Part model, mm, in its own coordinate system. A direction names the side the tool comes from. Coordinates: 2 decimals unless noted, no trailing zeros. Loops run counter-clockwise (first coordinate to the right, second up) from the corner with the lowest first, then second, coordinate; pieces in that order, holes last. Notation, with made-up numbers: (-31.5, 68) - (-23.5, 68) arc R32 ccw to (-23.5, 106) - close; hole circle Ø3 at (31.25, 55.5). An arc over 180 degrees is marked (long way). Use a Markdown table: item, result. Add a question column.
1. Band-saw the part on A-A, the plane y = -11. Give the cut face in (x, z).
2. Band-saw the part on B-B, the plane x = 8.5. Count the separate pieces of the cut face and the enclosed holes in it, plus the area to 3 significant figures.
3. Pull direction Z, two halves, no side cores. Call faces 4 (the flat face through (4, -46.7, 0)), 5 (the cylindrical face through (-19.458, -53.208, -6.128)), 6 (the flat face through (14, -59.9, 14)): pulls with the +Z half, pulls with the -Z half, needs draft (parallel to the pull), parting line crosses it, or undercut.
4. Wall check: probe 1 along Z at (x, y) = (0, -55.5); probe 2 along Y at (x, z) = (-11.5, -14.5); probe 3 along X at (y, z) = (-54.5, 17.5). Give the ranges that are in metal, low to high. Write a range as [from, to].
5. Drop flat-ended pins along their axis: pin 1 (2.5 mm diameter, centred on x = 14.5, z = 8, fed in from -Y); pin 2 (2 mm diameter, centred on x = 11, z = 15.5, fed in from +Y); pin 3 (1 mm diameter, centred on x = -18, y = -55.5, fed in from +Z). Give the stop position or say it passes through.
6. Band-saw the part on D-D, the plane y = -42. Give the cut face in (x, z).
7. 3-axis set-ups, long thin cutter, end or side, ignore diameter. For faces 1 (the flat face through (0, -47.4, 18)), 2 (the cylindrical face through (0, -62, 2)), 3 (the cylindrical face through (8.87, -45.94, 6.94)): which of +Z, -Z, +X, -X, +Y, -Y reach the whole face in a straight line?
from build123d import *

# Parameters (mm, degrees)
SKETCH2_R          = 4.25
CUT_EXTRUDE1_DEPTH = 54.622383424
CHAMFER1_SIZE      = 0.5
CIRPATTERN1_START  = -59.4
CIRPATTERN1_DEPTH  = 12


# Read off the part's stored shape, not the designer's step: CirPattern1
with BuildPart() as part:
    # Sketch1 → Revolve1 (revolve)
    with BuildSketch(Plane.XY, mode=Mode.PRIVATE) as revolve1_sk:
        with BuildLine():
            Line((0, 0), (0, -77.5))
            Line((0, -77.5), (2, -77.5))
            Line((2, -77.5), (2, -46.7))
            Line((2, -46.7), (18.9, -46.7))
            Line((18.9, -46.7), (18.9, -59.9))
            Line((18.9, -59.9), (20.4, -59.9))
            Line((20.4, -59.9), (20.4, -46.7))
            ThreePointArc((20.4, -46.7), (19.960660172, -45.639339828), (18.9, -45.2))
            Line((18.9, -45.2), (6, -45.2))
            ThreePointArc((6, -45.2), (5.292893219, -44.907106781), (5, -44.2))
            Line((5, -44.2), (5, -39.7))
            ThreePointArc((5, -39.7), (4.853553391, -39.346446609), (4.5, -39.2))
            Line((4.5, -39.2), (2, -39.2))
            Line((2, -39.2), (2, 0))
            Line((2, 0), (0, 0))
        make_face()
    revolve(revolve1_sk.sketch.rotate(Axis((0, 0, 0), (0, -1, 0)), 180), axis=Axis((0, 0, 0), (0, -1, 0)))

    # Sketch2 → Cut-Extrude1 (cut, through all)
    with BuildSketch(Plane(origin=(0, -45.2, 0), x_dir=(1, 0, 0), z_dir=(0, 1, 0))):
        with Locations(Location((5.5, 9.526279442, 0), (0, 0, 180))):
            Circle(SKETCH2_R)
        with Locations(Location((11, 0, 0), (0, 0, 180))):
            Circle(SKETCH2_R)
        with Locations(Location((5.5, -9.526279442, 0), (0, 0, 180))):
            Circle(SKETCH2_R)
        with Locations(Location((-5.5, -9.526279442, 0), (0, 0, 180))):
            Circle(SKETCH2_R)
        with Locations(Location((-11, 0, 0), (0, 0, 180))):
            Circle(SKETCH2_R)
        with Locations(Location((-5.5, 9.526279442, 0), (0, 0, 180))):
            Circle(SKETCH2_R)
    extrude(amount=-CUT_EXTRUDE1_DEPTH, mode=Mode.SUBTRACT)

    # Chamfer1
    chamfer1_edges = [part.edges().sort_by_distance(p)[0] for p in [
        (2, 0, 0),
        (2, -77.5, 0),
    ]]
    chamfer(chamfer1_edges, length=CHAMFER1_SIZE)

    # CirPattern1 outline → CirPattern1 (add)
    with BuildSketch(Plane(origin=(0, 0, 0), x_dir=(1, 0, 0), z_dir=(0, 1, 0)).offset(CIRPATTERN1_START)):
        with BuildLine():
            ThreePointArc((-3.9, -18.493242009), (0, -18.9), (3.9, -18.493242009))
            Line((3.9, -18.493242009), (3.9, -17.3))
            Line((3.9, -17.3), (-3.9, -17.3))
            Line((-3.9, -17.3), (-3.9, -18.493242009))
        make_face()
        with BuildLine():
            Line((5.272500925, -16.932239485), (5.86912193, -17.965617378))
            ThreePointArc((5.86912193, -17.965617378), (9.45, -16.367880131), (12.624120079, -14.065617378))
            Line((12.624120079, -14.065617378), (12.027499075, -13.032239485))
            Line((12.027499075, -13.032239485), (5.272500925, -16.932239485))
        make_face()
        with BuildLine():
            ThreePointArc((-12.624120079, -14.065617378), (-9.45, -16.367880131), (-5.86912193, -17.965617378))
            Line((-5.86912193, -17.965617378), (-5.272500925, -16.932239485))
            Line((-5.272500925, -16.932239485), (-12.027499075, -13.032239485))
            Line((-12.027499075, -13.032239485), (-12.624120079, -14.065617378))
        make_face()
        with BuildLine():
            Line((13.032239485, -12.027499075), (14.065617378, -12.624120079))
            ThreePointArc((14.065617378, -12.624120079), (16.367880131, -9.45), (17.965617378, -5.86912193))
            Line((17.965617378, -5.86912193), (16.932239485, -5.272500925))
            Line((16.932239485, -5.272500925), (13.032239485, -12.027499075))
        make_face()
        with BuildLine():
            ThreePointArc((-17.965617378, -5.86912193), (-16.367880131, -9.45), (-14.065617378, -12.624120079))
            Line((-14.065617378, -12.624120079), (-13.032239485, -12.027499075))
            Line((-13.032239485, -12.027499075), (-16.932239485, -5.272500925))
            Line((-16.932239485, -5.272500925), (-17.965617378, -5.86912193))
        make_face()
        with BuildLine():
            Line((17.3, -3.9), (18.493242009, -3.9))
            ThreePointArc((18.493242009, -3.9), (18.9, 0), (18.493242009, 3.9))
            Line((18.493242009, 3.9), (17.3, 3.9))
            Line((17.3, 3.9), (17.3, -3.9))
        make_face()
        with BuildLine():
            ThreePointArc((-18.493242009, 3.9), (-18.9, 0), (-18.493242009, -3.9))
            Line((-18.493242009, -3.9), (-17.3, -3.9))
            Line((-17.3, -3.9), (-17.3, 3.9))
            Line((-17.3, 3.9), (-18.493242009, 3.9))
        make_face()
        with BuildLine():
            ThreePointArc((-14.065617378, 12.624120079), (-16.367880131, 9.45), (-17.965617378, 5.86912193))
            Line((-17.965617378, 5.86912193), (-16.932239485, 5.272500925))
            Line((-16.932239485, 5.272500925), (-13.032239485, 12.027499075))
            Line((-13.032239485, 12.027499075), (-14.065617378, 12.624120079))
        make_face()
        with BuildLine():
            Line((16.932239485, 5.272500925), (17.965617378, 5.86912193))
            ThreePointArc((17.965617378, 5.86912193), (16.367880131, 9.45), (14.065617378, 12.624120079))
            Line((14.065617378, 12.624120079), (13.032239485, 12.027499075))
            Line((13.032239485, 12.027499075), (16.932239485, 5.272500925))
        make_face()
        with BuildLine():
            ThreePointArc((-5.86912193, 17.965617378), (-9.45, 16.367880131), (-12.624120079, 14.065617378))
            Line((-12.624120079, 14.065617378), (-12.027499075, 13.032239485))
            Line((-12.027499075, 13.032239485), (-5.272500925, 16.932239485))
            Line((-5.272500925, 16.932239485), (-5.86912193, 17.965617378))
        make_face()
        with BuildLine():
            Line((12.027499075, 13.032239485), (12.624120079, 14.065617378))
            ThreePointArc((12.624120079, 14.065617378), (9.45, 16.367880131), (5.86912193, 17.965617378))
            Line((5.86912193, 17.965617378), (5.272500925, 16.932239485))
            Line((5.272500925, 16.932239485), (12.027499075, 13.032239485))
        make_face()
        with BuildLine():
            ThreePointArc((3.9, 18.493242009), (0, 18.9), (-3.9, 18.493242009))
            Line((-3.9, 18.493242009), (-3.9, 17.3))
            Line((-3.9, 17.3), (3.9, 17.3))
            Line((3.9, 17.3), (3.9, 18.493242009))
        make_face()
    extrude(amount=CIRPATTERN1_DEPTH)


solid = part.part
Geometry check:
| question | item | result |
|---|---|---|
| 1 | outline | circle Ø4 at (0, 0) |
| 2 | separate pieces | 4 |
| 2 | enclosed holes | 0 |
| 2 | area | 114 mm^2 |
| 3 | face 4 | undercut |
| 3 | face 5 | parting line crosses it |
| 3 | face 6 | needs draft |
| 4 | probe 1 | z = [-20.4, -17.3], [-2, 2], [17.3, 20.4] |
| 4 | probe 2 | y = [-59.4, -47.4], [-46.7, -45.2] |
| 4 | probe 3 | x = [-10.48, -5.6], [-3.9, 3.9], [5.6, 10.48] |
| 5 | pin 1 | stops at y = -59.4 |
| 5 | pin 2 | stops at y = -45.2 |
| 5 | pin 3 | stops at z = 10.48 |
| 6 | outline | circle Ø10 at (0, 0) |
| 7 | face 1 | none |
| 7 | face 2 | -Y |
| 7 | face 3 | +Y, -Y |
